Autodesk Inventor part; units mm, degrees
ref_plane "YZ Plane" through (0, 0, 0) normal (1, 0, 0) x (0, 1, 0)
ref_plane "XZ Plane" through (0, 0, 0) normal (0, 1, 0) x (-1, 0, 0)
ref_plane "XY Plane" through (0, 0, 0) normal (0, 0, 1) x (1, 0, 0)
sketch "Sketch1" plane through (0, 0, 0) normal (1, 0, 0) x (0, 1, 0)
  line L0 (-7.5, 7.5) -> (7.5, 7.5)
  line L1 (7.5, 7.5) -> (7.5, -7.5)
  line L2 (7.5, -7.5) -> (-7.5, -7.5)
  line L3 (-7.5, -7.5) -> (-7.5, 7.5)
  line L4 (-7.5, 7.5) -> (7.5, -7.5) construction
  line L5 (7.5, 7.5) -> (-7.5, -7.5) construction
  line L6 (-6.5, 6.5) -> (6.5, 6.5)
  line L7 (6.5, 6.5) -> (6.5, -6.5)
  line L8 (6.5, -6.5) -> (-6.5, -6.5)
  line L9 (-6.5, -6.5) -> (-6.5, 6.5)
  line L10 (-6.5, 6.5) -> (6.5, -6.5) construction
  line L11 (6.5, 6.5) -> (-6.5, -6.5) construction
  point P0 (0, 0)
  dimension "d0" = 15
  dimension "d1" = 15
  dimension "d2" = 13
  dimension "d3" = 13
extrude "Extrusion1" add sketch "Sketch1" along normal blind 110
sketch "Sketch2" plane through (0, 7.5, 7.5) normal (0, 1, 0) x (1, 0, 0)
  line L0 (0, 7.5) -> (4, 7.5)
  circle A0 centre (4, 7.5) radius 1.5
  dimension "d6" = 4
  dimension "d7" = 3
extrude "Extrusion2" cut sketch "Sketch2" against normal through all
sketch "Sketch3" plane through (0, -7.5, -7.5) normal (0, -1, 0) x (1, 0, 0)
  line L0 (110, 1) -> (110, 14)
  line L1 (110, 7.5) -> (105, 7.5)
  circle A0 centre (105, 7.5) radius 1.5
  point P0 (0, 7.5)
  dimension "d10" = 5
  dimension "d11" = 3
extrude "Extrusion3" cut sketch "Sketch3" against normal up to next
properties part number "front_arm_rect" material "Aluminum 6061"
Input: part model. Units: mm. Frame: model coordinates. A direction names the side the tool comes from. Give positions to 0.01 mm unless a question says otherwise; leave off trailing zeros. Order: outer loops, then holes, each group sorted by start corner. A loop starts at its lowest first (then second) coordinate and runs counter-clockwise, first axis right, second up. Notation, with made-up numbers: (59, -30.75) - (107, -30.75) arc R29 ccw to (107, -2.75) - close; hole circle Ø2 at (48, -15.75). An arc over 180 degrees is marked (long way). Put each result on its own line as item: value.
Item 1: Section query D-D, the plane x = 40.5. Return loops of the section in (y, z), then the cut area to 3 significant figures.
Found:
outline: (-7.5, -7.5) - (7.5, -7.5) - (7.5, 7.5) - (-7.5, 7.5) - close; hole (-6.5, -6.5) - (6.5, -6.5) - (6.5, 6.5) - (-6.5, 6.5) - close
area: 56.0 mm^2
Item 2: Ray query, L1, parallel to Z at x = 104.5, y = -0.25; L2, parallel to Z at x = 4, y = -7.15. Return the intervals inside material, ascending. Write a range as from..to.
Found:
L1: z = -7.5..-6.5, 6.5..7.5
L2: z = -7.5..-1.5, 1.5..7.5
Item 3: Access query for faces 4 (the cylindrical face through (103.5, -7.01, 0.07)), 5 (the flat face through (54, 6.5, 0)), 6 (the flat face through (110, -7, 0)). Directions: +Z, -Z, +X, -X, +Y, -Y. A direction counts if a zero-diameter tool reaches every point of the face in a straight line with its end or side. Return the directions, or none.
Found:
face 4: -Y
face 5: +X, -X
face 6: +Z, -Z, +X, +Y, -Y
Item 4: Section query B-B, the plane y = -1.5. Return loops of the section in (x, z).
Found:
outline: (0, -7.5) - (110, -7.5) - (110, -6.5) - (0, -6.5) - close; (0, 6.5) - (110, 6.5) - (110, 7.5) - (0, 7.5) - close
Item 5: Section query A-A, the plane z = 0. Return loops of the section in (x, y).
Found:
outline: (0, -7.5) - (2.5, -7.5) - (2.5, -6.5) - (0, -6.5) - close; (0, 6.5) - (2.5, 6.5) - (2.5, 7.5) - (0, 7.5) - close; (5.5, -7.5) - (103.5, -7.5) - (103.5, -6.5) - (5.5, -6.5) - close; (5.5, 6.5) - (110, 6.5) - (110, 7.5) - (5.5, 7.5) - close; (106.5, -7.5) - (110, -7.5) - (110, -6.5) - (106.5, -6.5) - close
Item 6: Draft query along X for faces 1 (the flat face through (0, -7, 0)), 2 (the cylindrical face through (5.386, 7.007, 0.575)), 3 (the flat face through (54, -7.5, 0)). Return one class per face: +X half, -X half, draft (parallel to the pull), parting line (faces both ways), or undercut.
Found:
face 1: -X half
face 2: undercut
face 3: draft
Item 7: Section query C-C, the plane x = 4. Return loops of the section in (y, z), then the cut area to 3 significant figures.
Found:
outline: (-7.5, -7.5) - (7.5, -7.5) - (7.5, -1.5) - (6.5, -1.5) - (6.5, -6.5) - (-6.5, -6.5) - (-6.5, -1.5) - (-7.5, -1.5) - close; (-7.5, 1.5) - (-6.5, 1.5) - (-6.5, 6.5) - (6.5, 6.5) - (6.5, 1.5) - (7.5, 1.5) - (7.5, 7.5) - (-7.5, 7.5) - close
area: 50.0 mm^2
